CAD build for the part. Positions are in the model's coordinates, mm. A direction names the side the tool comes from. Give positions to 0.01 mm unless a question says otherwise; leave off trailing zeros. Order: outer loops, then holes, each group sorted by start corner. A loop starts at its lowest first (then second) coordinate and runs counter-clockwise, first axis right, second up. Notation, with made-up numbers: M -34.75,79.5 L -6.75,79.5 A15 ccw -6.75,93.5 Z; hole C 15.25,30 d4. An arc over 180 degrees is marked long. Put each result on its own line as item: value. Start each with the question number.
1) Two-plate mould, pull along X, no slides. Class faces 1 (the face through (-24.223, -6, 2)), 2 (the face through (1, -17, 0)), 3 (the face through (23.184, -25.344, 1.972)): released by +X, released by -X, zero draft, split by the parting line, or undercut.
2) Pin check, flat tip, straight feed: pin 1 (2 mm diameter, centred on x = 2, z = 2.5, fed in from +Y). Stop position of the tip, or through.
3) Cut at B-B (y = -9). Write the cut outline in (x, z).
4) Cut at A-A (x = 21). Write the cut outline in (y, z), and give its area (3 significant figures).
5) Cut at D-D (x = 11). Write the cut outline in (y, z), and give its area (3 significant figures).
6) Drill centre lines: line 1 (X direction, y = 11, z = 2.6); line 2 (X direction, y = 14.5, z = 1.9); line 3 (Y direction, x = -19, z = 2.8). Where is each one in solid material? Low to high. Write a range as [from, to].
7) Tool access for faces 4 (the face through (1, -17, 4)), 5 (the face through (1, -12.202, 2)): list every direction of +Z, -Z, +X, -X, +Y, -Y with a clear straight run to the whole face (end or side of a thin tool).
8) Cut at C-C (z = 0.8). Write the cut outline in (x, y), and give its area (3 significant figures).
```python
from build123d import *

# Parameters (mm, degrees)
SKETCH_1_R          = 2
EXTRUDE_1_DEPTH     = 4
SKETCH_2_W          = 21
SKETCH_2_H          = 31.756996305
CUT_EXTRUDE_1_DEPTH = 4


with BuildPart() as part:
    # 草图1 → 凸台-拉伸1 (new body)
    with BuildSketch(Plane.XY):
        Polygon((-24.223404255, 19.554868645), (-24.223404255, -31.445131355), (-24.223404255, -31.945131355), (26.776595745, -31.945131355), (26.776595745, -31.445131355), (26.776595745, 19.554868645), align=None)
        with Locations((-18.723404255, -25.945131355)):
            Circle(SKETCH_1_R, mode=Mode.SUBTRACT)
        with Locations((21.276595745, -25.945131355)):
            Circle(SKETCH_1_R, mode=Mode.SUBTRACT)
        with Locations((-18.723404255, 14.054868645)):
            Circle(SKETCH_1_R, mode=Mode.SUBTRACT)
        with Locations((21.276595745, 14.054868645)):
            Circle(SKETCH_1_R, mode=Mode.SUBTRACT)
    extrude(amount=EXTRUDE_1_DEPTH)

    # 草图2 → 切除-拉伸1 (cut)
    with BuildSketch(Plane.XY.offset(4)):
        with Locations((1.276595745, 3.676370493)):
            Rectangle(SKETCH_2_W, SKETCH_2_H)
    extrude(amount=-CUT_EXTRUDE_1_DEPTH, mode=Mode.SUBTRACT)


solid = part.part
```
Solution:
1. face 1: released by -X
1. face 2: zero draft
1. face 3: undercut
2. pin 1: y = -12.2
3. outline: M -24.22,0 L -9.22,0 L -9.22,4 L -24.22,4 Z; M 11.78,0 L 26.78,0 L 26.78,4 L 11.78,4 Z
4. outline: M -31.95,0 L -27.93,0 L -27.93,4 L -31.95,4 Z; M -23.96,0 L 12.07,0 L 12.07,4 L -23.96,4 Z; M 16.04,0 L 19.55,0 L 19.55,4 L 16.04,4 Z
4. area: 174 mm²
5. outline: M -31.95,0 L -12.2,0 L -12.2,4 L -31.95,4 Z
5. area: 79.0 mm²
6. line 1: [-24.22, -9.22], [11.78, 26.78]
6. line 2: [-24.22, -20.67], [-16.77, -9.22], [11.78, 19.33], [23.23, 26.78]
6. line 3: [-31.95, -27.93], [-23.96, 12.07], [16.04, 19.55]
7. face 4: +Z, +X, -X, +Y, -Y
7. face 5: +Z, -Z, +Y
8. outline: M -24.22,-31.95 L 26.78,-31.95 L 26.78,19.55 L 11.78,19.55 L 11.78,-12.2 L -9.22,-12.2 L -9.22,19.55 L -24.22,19.55 Z; hole C -18.72,-25.95 d4; hole C -18.72,14.05 d4; hole C 21.28,-25.95 d4; hole C 21.28,14.05 d4
8. area: 1,910 mm²
